from build123d import *

# Parameters (mm, degrees)
EXTRUDE1_DEPTH          = 7.9375
SKETCH13_R              = 6.35
EXTRUDE3_DEPTH          = 1.5875
SKETCH2_OUTSIDE_W       = 63.61
SKETCH2_OUTSIDE_H       = 63.61
SKETCH2_OUTSIDE_R       = 4.7625
CUT_EXTRUDE1_DEPTH      = 12.985362166
CUT_EXTRUDE1_DRAFT      = -60
SKETCH14_R              = 1.8161
BOSS_EXTRUDE1_DEPTH     = 12.7
MIRROR1_COPY_1_SKETCH_W = 63.61
MIRROR1_COPY_1_SKETCH_H = 63.61
MIRROR1_COPY_1_SKETCH_R = 4.7625
MIRROR1_COPY_1_DEPTH    = 12.985362166
MIRROR1_COPY_1_DRAFT    = -60
SKETCH15_R              = 1.8161
BOSS_EXTRUDE2_DEPTH     = 254
MIRROR2_COPY_1_SKETCH_W = 63.61
MIRROR2_COPY_1_SKETCH_H = 63.61
MIRROR2_COPY_1_SKETCH_R = 4.7625
MIRROR2_COPY_1_DEPTH    = 12.985362166
MIRROR2_COPY_1_DRAFT    = -60
MIRROR2_COPY_2_DEPTH    = 7.9375
MIRROR2_COPY_3_SKETCH_R = 6.35
MIRROR2_COPY_3_DEPTH    = 1.5875
MIRROR2_COPY_4_SKETCH_R = 1.8161
MIRROR2_COPY_4_DEPTH    = 12.7
MIRROR2_COPY_5_SKETCH_W = 63.61
MIRROR2_COPY_5_SKETCH_H = 63.61
MIRROR2_COPY_5_SKETCH_R = 4.7625
MIRROR2_COPY_5_DEPTH    = 12.985362166
MIRROR2_COPY_5_DRAFT    = -60
SKETCH16_R              = 1.8161
BOSS_EXTRUDE3_DEPTH     = 25.4
SKETCH4_R               = 1.8161
BOSS_EXTRUDE4_DEPTH     = 25.4


with BuildPart() as part:
    # Sketch1 → Extrude1 (new body)
    with BuildSketch(Plane.XY):
        Polygon((0, 5.499261314), (-4.7625, 2.749630657), (-4.7625, -2.749630657), (0, -5.499261314), (4.7625, -2.749630657), (4.7625, 2.749630657), align=None)
    extrude1 = extrude(amount=-EXTRUDE1_DEPTH)

    # Sketch13 → Extrude3 (add)
    with BuildSketch(Plane(origin=(0, 0, -7.9375), x_dir=(-1, 0, 0), z_dir=(0, 0, -1))):
        Circle(SKETCH13_R)
    extrude3 = extrude(amount=-EXTRUDE3_DEPTH)


with BuildPart() as cut_extrude1_tool:
    # Sketch2 outside → Cut-Extrude1 (with draft: the straight prism first)
    with BuildSketch(Plane.XY):
        Rectangle(SKETCH2_OUTSIDE_W, SKETCH2_OUTSIDE_H)
        Circle(SKETCH2_OUTSIDE_R, mode=Mode.SUBTRACT)
    extrude(amount=-CUT_EXTRUDE1_DEPTH)
    # Cut-Extrude1: the draft: its side faces are tilted about the plane it starts from
    cut_extrude1_sides = [cut_extrude1_tool.faces().sort_by_distance(p)[0] for p in [
        (0, -31.805, -6.492681083),
        (31.805, 0, -6.492681083),
        (0, 31.805, -6.492681083),
        (-31.805, 0, -6.492681083),
        (-4.7625, 0, -6.492681083),
    ]]
    draft(cut_extrude1_sides, Plane.XY, CUT_EXTRUDE1_DRAFT)


with BuildPart() as part_1:
    add(part.part)

    # Cut-Extrude1: cut by cut_extrude1_tool
    add(cut_extrude1_tool.part, mode=Mode.SUBTRACT)

    # Sketch14 → Boss-Extrude1 (add)
    with BuildSketch(Plane(origin=(0, 0, -7.9375), x_dir=(-1, 0, 0), z_dir=(0, 0, -1))):
        Circle(SKETCH14_R)
    boss_extrude1 = extrude(amount=BOSS_EXTRUDE1_DEPTH)

    # Mirror1: Extrude1, Extrude3, Boss-Extrude1 across plane
    add(extrude1.mirror(Plane(origin=(0, 0, -20.6375), x_dir=(1, 0, 0), z_dir=(0, 0, -1))))
    add(extrude3.mirror(Plane(origin=(0, 0, -20.6375), x_dir=(1, 0, 0), z_dir=(0, 0, -1))))
    add(boss_extrude1.mirror(Plane(origin=(0, 0, -20.6375), x_dir=(1, 0, 0), z_dir=(0, 0, -1))))


with BuildPart() as mirror1_copy_1_tool:
    # Mirror1 copy 1 sketch → Mirror1 copy 1 (with draft: the straight prism first)
    with BuildSketch(Plane(origin=(0, 0, -41.275), x_dir=(1, 0, 0), z_dir=(0, 0, -1))):
        Rectangle(MIRROR1_COPY_1_SKETCH_W, MIRROR1_COPY_1_SKETCH_H)
        Circle(MIRROR1_COPY_1_SKETCH_R, mode=Mode.SUBTRACT)
    extrude(amount=-MIRROR1_COPY_1_DEPTH)
    # Mirror1 copy 1: the draft: its side faces are tilted about the plane it starts from
    mirror1_copy_1_sides = [mirror1_copy_1_tool.faces().sort_by_distance(p)[0] for p in [
        (0, -31.805, -34.782318917),
        (31.805, 0, -34.782318917),
        (0, 31.805, -34.782318917),
        (-31.805, 0, -34.782318917),
        (-4.7625, 0, -34.782318917),
    ]]
    draft(mirror1_copy_1_sides, Plane(origin=(0, 0, -41.275), x_dir=(1, 0, 0), z_dir=(0, 0, -1)), MIRROR1_COPY_1_DRAFT)


with BuildPart() as part_2:
    add(part_1.part)

    # Mirror1 copy 1: cut by mirror1_copy_1_tool
    add(mirror1_copy_1_tool.part, mode=Mode.SUBTRACT)

    # Sketch15 → Boss-Extrude2 (add)
    with BuildSketch(Plane(origin=(0, 0, -41.275), x_dir=(-1, 0, 0), z_dir=(0, 0, -1))):
        Circle(SKETCH15_R)
    boss_extrude2 = extrude(amount=BOSS_EXTRUDE2_DEPTH)

    # Mirror2: Extrude1, Extrude3, Boss-Extrude1, Boss-Extrude2 across plane
    add(extrude1.mirror(Plane(origin=(0, 0, -295.275), x_dir=(1, 0, 0), z_dir=(0, 0, -1))))
    add(extrude3.mirror(Plane(origin=(0, 0, -295.275), x_dir=(1, 0, 0), z_dir=(0, 0, -1))))
    add(boss_extrude1.mirror(Plane(origin=(0, 0, -295.275), x_dir=(1, 0, 0), z_dir=(0, 0, -1))))
    add(boss_extrude2.mirror(Plane(origin=(0, 0, -295.275), x_dir=(1, 0, 0), z_dir=(0, 0, -1))))


with BuildPart() as mirror2_copy_1_tool:
    # Mirror2 copy 1 sketch → Mirror2 copy 1 (with draft: the straight prism first)
    with BuildSketch(Plane(origin=(0, 0, -590.55), x_dir=(1, 0, 0), z_dir=(0, 0, -1))):
        Rectangle(MIRROR2_COPY_1_SKETCH_W, MIRROR2_COPY_1_SKETCH_H)
        Circle(MIRROR2_COPY_1_SKETCH_R, mode=Mode.SUBTRACT)
    extrude(amount=-MIRROR2_COPY_1_DEPTH)
    # Mirror2 copy 1: the draft: its side faces are tilted about the plane it starts from
    mirror2_copy_1_sides = [mirror2_copy_1_tool.faces().sort_by_distance(p)[0] for p in [
        (0, -31.805, -584.057318917),
        (31.805, 0, -584.057318917),
        (0, 31.805, -584.057318917),
        (-31.805, 0, -584.057318917),
        (-4.7625, 0, -584.057318917),
    ]]
    draft(mirror2_copy_1_sides, Plane(origin=(0, 0, -590.55), x_dir=(1, 0, 0), z_dir=(0, 0, -1)), MIRROR2_COPY_1_DRAFT)


with BuildPart() as part_3:
    add(part_2.part)

    # Mirror2 copy 1: cut by mirror2_copy_1_tool
    add(mirror2_copy_1_tool.part, mode=Mode.SUBTRACT)

    # Mirror2 copy 2 sketch → Mirror2 copy 2 (add)
    with BuildSketch(Plane.XY.offset(-549.275)):
        Polygon((0, 5.499261314), (-4.7625, 2.749630657), (-4.7625, -2.749630657), (0, -5.499261314), (4.7625, -2.749630657), (4.7625, 2.749630657), align=None)
    extrude(amount=-MIRROR2_COPY_2_DEPTH)

    # Mirror2 copy 3 sketch → Mirror2 copy 3 (add)
    with BuildSketch(Plane(origin=(0, 0, -557.2125), x_dir=(-1, 0, 0), z_dir=(0, 0, -1))):
        Circle(MIRROR2_COPY_3_SKETCH_R)
    extrude(amount=-MIRROR2_COPY_3_DEPTH)

    # Mirror2 copy 4 sketch → Mirror2 copy 4 (add)
    with BuildSketch(Plane(origin=(0, 0, -557.2125), x_dir=(-1, 0, 0), z_dir=(0, 0, -1))):
        Circle(MIRROR2_COPY_4_SKETCH_R)
    extrude(amount=MIRROR2_COPY_4_DEPTH)


with BuildPart() as mirror2_copy_5_tool:
    # Mirror2 copy 5 sketch → Mirror2 copy 5 (with draft: the straight prism first)
    with BuildSketch(Plane.XY.offset(-549.275)):
        Rectangle(MIRROR2_COPY_5_SKETCH_W, MIRROR2_COPY_5_SKETCH_H)
        Circle(MIRROR2_COPY_5_SKETCH_R, mode=Mode.SUBTRACT)
    extrude(amount=-MIRROR2_COPY_5_DEPTH)
    # Mirror2 copy 5: the draft: its side faces are tilted about the plane it starts from
    mirror2_copy_5_sides = [mirror2_copy_5_tool.faces().sort_by_distance(p)[0] for p in [
        (0, -31.805, -555.767681083),
        (31.805, 0, -555.767681083),
        (0, 31.805, -555.767681083),
        (-31.805, 0, -555.767681083),
        (-4.7625, 0, -555.767681083),
    ]]
    draft(mirror2_copy_5_sides, Plane.XY.offset(-549.275), MIRROR2_COPY_5_DRAFT)


with BuildPart() as part_4:
    add(part_3.part)

    # Mirror2 copy 5: cut by mirror2_copy_5_tool
    add(mirror2_copy_5_tool.part, mode=Mode.SUBTRACT)

    # Sketch16 → Boss-Extrude3 (add)
    with BuildSketch(Plane(origin=(0, 0, -590.55), x_dir=(-1, 0, 0), z_dir=(0, 0, -1))):
        Circle(SKETCH16_R)
    extrude(amount=BOSS_EXTRUDE3_DEPTH)

    # Sketch4 → Boss-Extrude4 (add)
    with BuildSketch(Plane.XY):
        with Locations(Location((0, 0, 0), (0, 0, 180))):
            Circle(SKETCH4_R)
    extrude(amount=BOSS_EXTRUDE4_DEPTH)


solid = part_4.part
Verification items for the finished model (mm, model axes). A direction names the side the tool comes from. Round coordinates to 2 decimals unless told otherwise and drop trailing zeros. Loops run counter-clockwise (first coordinate to the right, second up) from the corner with the lowest first, then second, coordinate; pieces in that order, holes last. Notation, with made-up numbers: M -25.75,-6 L 12.25,-6 A5 ccw 12.25,3 Z; hole C 2,11 d1. An arc over 180 degrees is marked long. Write each question's results on one line, items separated by ' | '.
1) Scan lines: L1, parallel to Z at x = -4.25, y = 3; L2, parallel to Y at x = 0.5, z = -281; L3, parallel to Y at x = -4.5, z = -4.5. Record each from-to range of solid material in increasing order. Write a range as from..to.
Checks:
L1: z = -590.3..-582.61, -557.21..-549.53, -41.02..-33.34, -7.94..-0.25 | L2: y = -1.75..1.75 | L3: y = -2.9..2.9
2) Gauge pin test, flat ends, axial feed: P1, Ø3, axis at y = 0.5, z = -67, coming from the +X side; P2, Ø4, axis at y = -3, z = -142, coming from the +X side; P3, Ø6, axis at y = 0, z = -589, coming from the -X side; P4, Ø5, axis at x = 2, y = 0.5, coming from the -Z side. Record the tip position at first contact, or that the pin passes through.
Checks:
P1: stops at x = 1.82 | P2: stops at x = 1.52 | P3: stops at x = -4.76 | P4: stops at z = -615.95
3) Access from +Z, -Z, +X, -X, +Y, -Y to the whole of each face (thin tool, end or side, straight path). Record for faces 5 (the cylindrical face through (1.38, -6.2, -7.15)), 6 (the flat face through (-1, 2, -33.338)).
Checks:
face 5: +Z, -Z | face 6: none
4) Section check A-A on z = -460.5. Record the boundary of the cut face in (x, y).
Checks:
outline: C 0,0 d3.63
5) Mould release check, pull along Z, two halves, no side actions. Record for faces 1 (the flat face through (2.4, 4.3, -6.35)), 2 (the flat face through (-1, 2, -7.938)), 3 (the flat face through (2.4, 4.3, -555.625)), 4 (the flat face through (2.4, 4.3, -584.2)): released by +Z, released by -Z, zero draft, split by the parting line, or undercut.
Checks:
face 1: released by +Z | face 2: undercut | face 3: undercut | face 4: released by -Z
